Study the drawing (mm; zero at the part's minimum x, y, z) and answer. Give positions to 0.01 mm unless a question says otherwise; leave off trailing zeros. Loops run counter-clockwise (first coordinate to the right, second up) from the corner with the lowest first, then second, coordinate; pieces in that order, holes last. Notation, with made-up numbers: (62, 47) - (75, 47) arc R21 cw to (75, 80) - close; hole circle Ø3 at (-36.75, -34.5). An arc over 180 degrees is marked (long way). Answer in a Markdown table with one row per item. Add a question column.
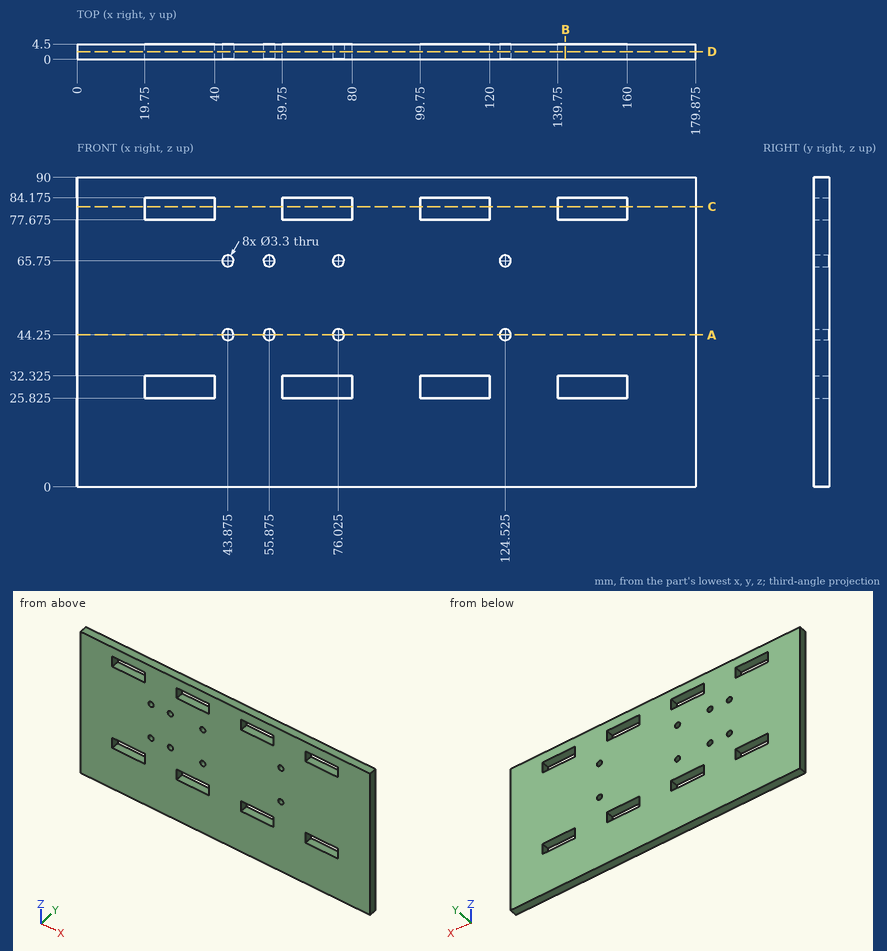
(1) A cutting plane is placed at C-C on z = 81.5. Determine the outline of the cut face in (x, y) (3 decimals).
(2) Find the intervals of material crossed by line 1 along Z through (x, y) = (36, 4.2) (3 decimals); line 2 along X through (y, z) = (1.45, 44.25) (3 decimals); line 3 along X through (y, z) = (3.75, 30.5) (3 decimals), in increasing order. Write a range as [from, to].
(3) A cutting plane is placed at D-D on y = 2.3. Give the number of separate pieces and of enclosed holes in the cut face, plus the area to 3 significant figures.
(4) A cutting plane is placed at B-B on x = 142. Determine the outline of the cut face in (y, z) (3 decimals).
(5) A cutting plane is placed at A-A on z = 44.25. Determine the outline of the cut face in (x, y) (3 decimals), plus the area to 3 significant figures.
(6) Given pin 1 Ø2 at (x, y) = (70, 3) entering from -Z, flat-ended and moving along its own axis, determine where the tip first touches the part or whether it passes through.
Evaluation:
| question | item | result |
|---|---|---|
| 1 | outline | (0, 0) - (19.75, 0) - (19.75, 4.5) - (0, 4.5) - close; (40, 0) - (59.75, 0) - (59.75, 4.5) - (40, 4.5) - close; (80, 0) - (99.75, 0) - (99.75, 4.5) - (80, 4.5) - close; (120, 0) - (139.75, 0) - (139.75, 4.5) - (120, 4.5) - close; (160, 0) - (179.875, 0) - (179.875, 4.5) - (160, 4.5) - close |
| 2 | line 1 | z = [0, 25.825], [32.325, 77.675], [84.175, 90] |
| 2 | line 2 | x = [0, 42.225], [45.525, 54.225], [57.525, 74.375], [77.675, 122.875], [126.175, 179.875] |
| 2 | line 3 | x = [0, 19.75], [40, 59.75], [80, 99.75], [120, 139.75], [160, 179.875] |
| 3 | separate pieces | 1 |
| 3 | enclosed holes | 16 |
| 3 | area | 15,100 mm² |
| 4 | outline | (0, 0) - (4.5, 0) - (4.5, 25.825) - (0, 25.825) - close; (0, 32.325) - (4.5, 32.325) - (4.5, 77.675) - (0, 77.675) - close; (0, 84.175) - (4.5, 84.175) - (4.5, 90) - (0, 90) - close |
| 5 | outline | (0, 0) - (42.225, 0) - (42.225, 4.5) - (0, 4.5) - close; (45.525, 0) - (54.225, 0) - (54.225, 4.5) - (45.525, 4.5) - close; (57.525, 0) - (74.375, 0) - (74.375, 4.5) - (57.525, 4.5) - close; (77.675, 0) - (122.875, 0) - (122.875, 4.5) - (77.675, 4.5) - close; (126.175, 0) - (179.875, 0) - (179.875, 4.5) - (126.175, 4.5) - close |
| 5 | area | 750 mm² |
| 6 | pin 1 | stops at z = 0 |
